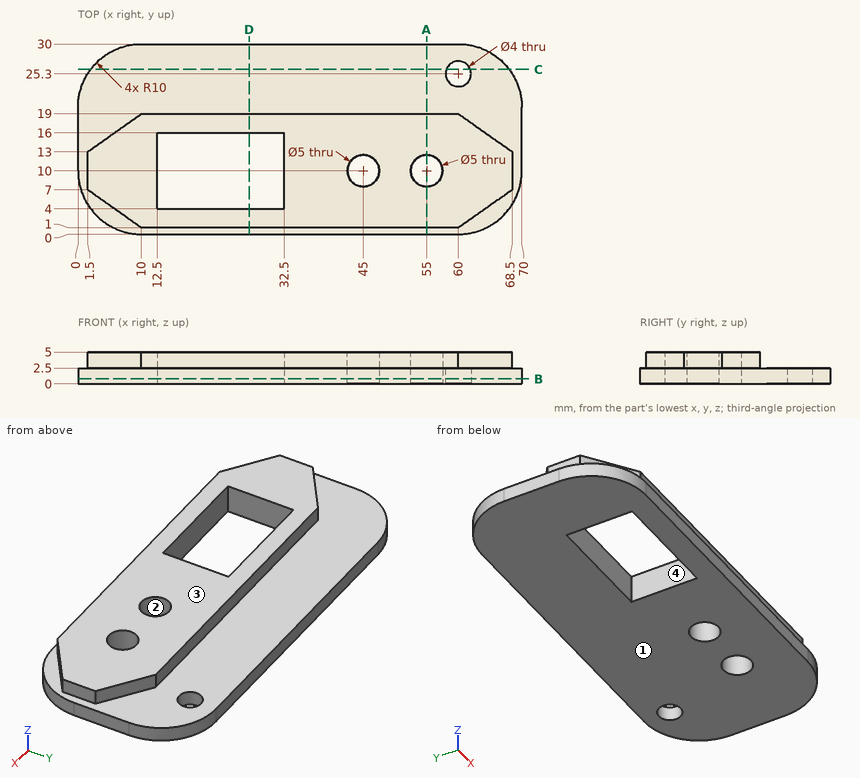
Geometry check sheet. Reference: drawing and pictorial views, mm from the part's lowest x, y, z. A direction names the side the tool comes from. Give positions to 0.01 mm unless a question says otherwise; leave off trailing zeros. Loops run counter-clockwise (first coordinate to the right, second up) from the corner with the lowest first, then second, coordinate; pieces in that order, holes last.
1. Section check B-B, the plane z = 0.8. Enter the section's corners in (x, y).
2. Mould release check, pull along X, two halves, no side actions. Record for the marked faces 1 and 2: released by +X, released by -X, zero draft, split by the parting line, or undercut.
3. Set-up check for the marked faces 3 and 4: record each of +Z, -Z, +X, -X, +Y, -Y from which the full face is reachable in a straight line by a thin tool's end or side.
4. Thickness scan on line 1 (X direction, y = 15.5, z = 2.2); line 2 (Y direction, x = 45, z = 2.8); line 3 (Y direction, x = 60, z = 1.4). Record the ranges inside material, lowest first.
5. Go/stop test with flat-tipped pins: pin 1 Ø3 at (y, z) = (4, 3) entering from +X; pin 2 Ø1.5 at (x, z) = (17, 1) entering from -Y; pin 3 Ø2.5 at (y, z) = (9, 3.5) entering from -X; pin 4 Ø2 at (x, z) = (29, 4) entering from +Y. Record where each tip stops, or that it passes through.
6. Section check A-A, the plane x = 55. Enter the section's corners in (y, z).
7. Section check C-C, the plane y = 26. Enter the section's corners in (x, z).
8. Section check D-D, the plane x = 27. Enter the section's corners in (y, z), then the cut area to 3 significant figures.
Geometry says:
1. outline: (0, 10) arc R10 ccw to (10, 0) - (60, 0) arc R10 ccw to (70, 10) - (70, 20) arc R10 ccw to (60, 30) - (10, 30) arc R10 ccw to (0, 20) - close; hole (12.5, 4) - (32.5, 4) - (32.5, 16) - (12.5, 16) - close; hole circle Ø5 at (45, 10); hole circle Ø5 at (55, 10); hole circle Ø4 at (60, 25.3)
2. face 1: zero draft
2. face 2: undercut
3. face 3: +Z, +X, -X, +Y, -Y
3. face 4: +Z, -Z
4. line 1: x = 0 to 12.5, 32.5 to 70
4. line 2: y = 1 to 7.5, 12.5 to 19
4. line 3: y = 0 to 23.3, 27.3 to 30
5. pin 1: stops at x = 68.89
5. pin 2: stops at y = 0
5. pin 3: stops at x = 0
5. pin 4: stops at y = 19
6. outline: (0, 0) - (7.5, 0) - (7.5, 5) - (1, 5) - (1, 2.5) - (0, 2.5) - close; (12.5, 0) - (30, 0) - (30, 2.5) - (19, 2.5) - (19, 5) - (12.5, 5) - close
7. outline: (2, 0) - (58.13, 0) - (58.13, 2.5) - (2, 2.5) - close; (61.87, 0) - (68, 0) - (68, 2.5) - (61.87, 2.5) - close
8. outline: (0, 0) - (4, 0) - (4, 5) - (1, 5) - (1, 2.5) - (0, 2.5) - close; (16, 0) - (30, 0) - (30, 2.5) - (19, 2.5) - (19, 5) - (16, 5) - close
8. area: 60.0 mm2
